```python
from build123d import *

# Parameters (mm, degrees)
SKETCH_R  = 1.55
PAD_DEPTH = 13


with BuildPart() as part:
    # Sketch → Pad (new body)
    with BuildSketch(Plane.XY):
        with BuildLine():
            ThreePointArc((-30, 4.5), (-34.5, 0), (-30, -4.5))
            Line((-30, -4.5), (30, -4.5))
            ThreePointArc((30, -4.5), (34.5, 0), (30, 4.5))
            Line((30, 4.5), (-30, 4.5))
        make_face()
        with Locations((-30, 0)):
            Circle(SKETCH_R, mode=Mode.SUBTRACT)
        with Locations((30, 0)):
            Circle(SKETCH_R, mode=Mode.SUBTRACT)
        Circle(SKETCH_R, mode=Mode.SUBTRACT)
        with Locations((-15, 0)):
            Circle(SKETCH_R, mode=Mode.SUBTRACT)
        with Locations((15, 0)):
            Circle(SKETCH_R, mode=Mode.SUBTRACT)
    extrude(amount=PAD_DEPTH)


solid = part.part
```
Input: part model. Units: mm. Frame: model coordinates. Give positions to 0.01 mm unless a question says otherwise; leave off trailing zeros. Loops run counter-clockwise (first coordinate to the right, second up) from the corner with the lowest first, then second, coordinate; pieces in that order, holes last. Notation, with made-up numbers: M -6,51 L 30,51 A26 ccw 30,88 Z; hole C -25,-30.75 d6. An arc over 180 degrees is marked long. Answer as CSV lines item,"result". Start each with the question number.
1. Section D-D on y = 3.25. Return loops of the section in (x, z), plus the area to 3 significant figures.
2. Line query: L1, parallel to Y at x = 30, z = 10; L2, parallel to X at y = -0.25, z = 4; L3, parallel to X at y = 1.25, z = 3.5. Output: solid intervals per line, ascending.
3. Section B-B on y = -0.75. Return loops of the section in (x, z).
4. Pin query (flat end, axial travel): P1, Ø3, axis at x = 24.5, y = 0.5, coming from the -Z side. Return the tip coordinate at first contact, or that it passes through.
5. Section A-A on z = 3.25. Return loops of the section in (x, y), plus the area to 3 significant figures.
6. Pull-direction query (Y, two-part tool) for faces 1 (the face through (-28.568, -0.594, 6.409)), 2 (the face through (0, 4.5, 6)), 3 (the face through (34.5, -0.1, 6.4)); classes: released by +Y, released by -Y, zero draft, split by the parting line, or undercut.
7. Section C-C on x = -15. Return loops of the section in (y, z).
Computed values:
1,outline,"M -33.11,0 L 33.11,0 L 33.11,13 L -33.11,13 Z"
1,area,"861 mm²"
2,L1,"y = -4.5 to -1.55, 1.55 to 4.5"
2,L2,"x = -34.49 to -31.53, -28.47 to -16.53, -13.47 to -1.53, 1.53 to 13.47, 16.53 to 28.47, 31.53 to 34.49"
2,L3,"x = -34.32 to -30.92, -29.08 to -15.92, -14.08 to -0.92, 0.92 to 14.08, 15.92 to 29.08, 30.92 to 34.32"
3,outline,"M -34.44,0 L -31.36,0 L -31.36,13 L -34.44,13 Z; M -28.64,0 L -16.36,0 L -16.36,13 L -28.64,13 Z; M -13.64,0 L -1.36,0 L -1.36,13 L -13.64,13 Z; M 1.36,0 L 13.64,0 L 13.64,13 L 1.36,13 Z; M 16.36,0 L 28.64,0 L 28.64,13 L 16.36,13 Z; M 31.36,0 L 34.44,0 L 34.44,13 L 31.36,13 Z"
4,P1,"stops at z = 0"
5,outline,"M -30,-4.5 L 30,-4.5 A4.5 ccw 30,4.5 L -30,4.5 A4.5 ccw Z; hole C -30,0 d3.1; hole C -15,0 d3.1; hole C 0,0 d3.1; hole C 15,0 d3.1; hole C 30,0 d3.1"
5,area,"566 mm²"
6,face 1,"undercut"
6,face 2,"released by +Y"
6,face 3,"split by the parting line"
7,outline,"M -4.5,0 L -1.55,0 L -1.55,13 L -4.5,13 Z; M 1.55,0 L 4.5,0 L 4.5,13 L 1.55,13 Z"
